Verification items for this drawing (mm, ordinates from the low corner). A direction names the side the tool comes from. Round coordinates to 2 decimals unless told otherwise and drop trailing zeros. Order: outer loops, then holes, each group sorted by start corner. A loop starts at its lowest first (then second) coordinate and runs counter-clockwise, first axis right, second up. Notation, with made-up numbers: (-9, -9.75) -> (9, -9.75) arc R22 ccw to (9, -2.75) -> close; hole circle Ø6 at (87.5, 85). An arc over 180 degrees is marked (long way). Answer in a Markdown table with one row per item.
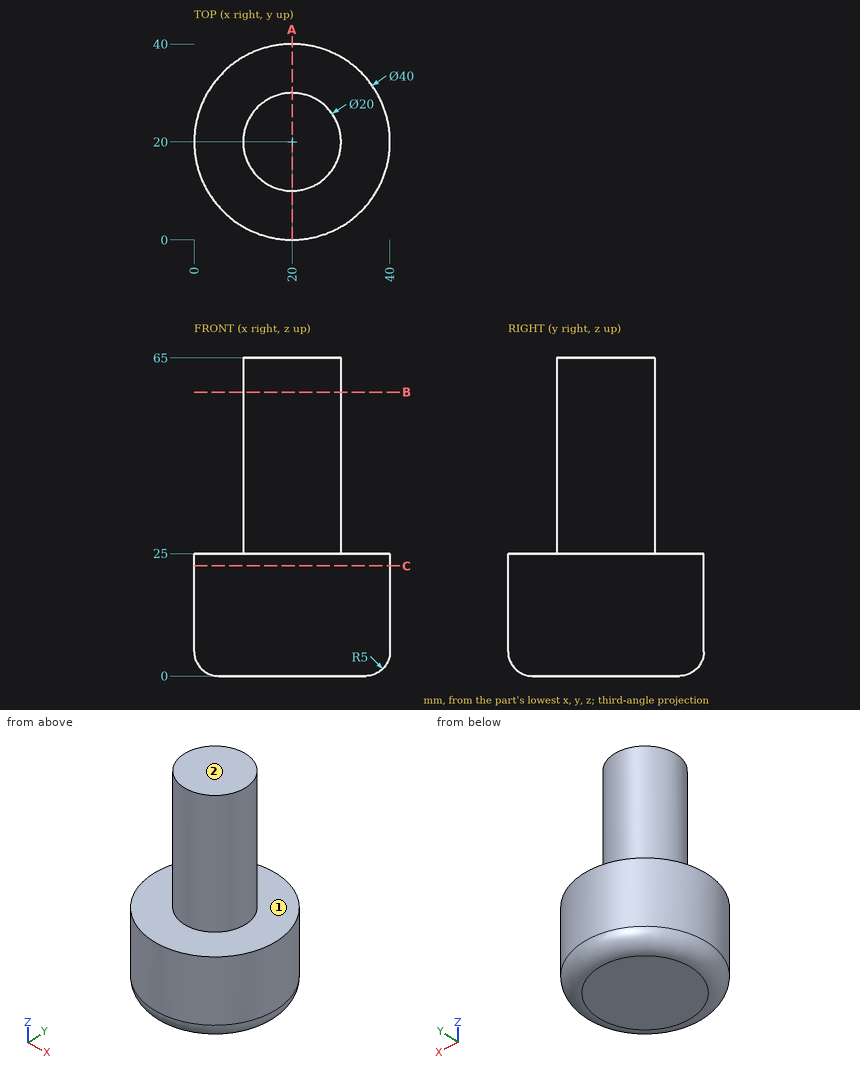
Item 1: Scan lines: line 1 (Z direction, x = 16.5, y = 5); line 2 (Y direction, x = 19.5, z = 35); line 3 (Y direction, x = 11.5, z = 5.5). Record each from-to range of solid material in increasing order. Write a range as [from, to].
Result sheet:
| item | result |
|---|---|
| line 1 | z = [0.02, 25] |
| line 2 | y = [10.01, 29.99] |
| line 3 | y = [1.9, 38.1] |
Item 2: Set-up check for the marked faces 1 and 2: record each of +Z, -Z, +X, -X, +Y, -Y from which the full face is reachable in a straight line by a thin tool's end or side.
Result sheet:
| item | result |
|---|---|
| face 1 | +Z |
| face 2 | +Z, +X, -X, +Y, -Y |
Item 3: Cross-section at B-B (z = 58). Record the boundary of the cut face in (x, y).
Result sheet:
| item | result |
|---|---|
| outline | circle Ø20 at (20, 20) |
Item 4: Depth check by flat-ended pin: P1, Ø8, axis at x = 12.5, z = 34, coming from the -Y side; P2, Ø3, axis at x = 21.5, z = 39.5, coming from the +Y side; P3, Ø5, axis at y = 11, z = 17, coming from the +X side. Enter the tip coordinate at first touch or a pass-through.
Result sheet:
| item | result |
|---|---|
| P1 | stops at y = 10.63 |
| P2 | stops at y = 30 |
| P3 | stops at x = 38.91 |
Item 5: Cross-section at A-A (x = 20). Record the boundary of the cut face in (y, z).
Result sheet:
| item | result |
|---|---|
| outline | (0, 5) arc R5 ccw to (5, 0) -> (35, 0) arc R5 ccw to (40, 5) -> (40, 25) -> (30, 25) -> (30, 65) -> (10, 65) -> (10, 25) -> (0, 25) -> close |
Item 6: Cross-section at C-C (z = 22.5). Record the boundary of the cut face in (x, y).
Result sheet:
| item | result |
|---|---|
| outline | circle Ø40 at (20, 20) |
